```python
from build123d import *

# Parameters (mm, degrees)
SKETCH_R        = 6.65
PAD_DEPTH       = 10
SKETCH001_R     = 2.55
POCKET_DEPTH    = 10
SKETCH002_W     = 3.1
SKETCH002_H     = 15.6
PAD001_DEPTH    = 16
SKETCH003_R     = 2.55
POCKET001_DEPTH = 65.851


with BuildPart() as part:
    # Sketch → Pad (new body)
    with BuildSketch(Plane.XY):
        with BuildLine():
            Line((0, -15.35), (19.8, -15.35))
            ThreePointArc((19.8, -15.35), (28.780256, -11.630256), (32.5, -2.65))
            Line((32.5, -2.65), (32.5, 2.65))
            ThreePointArc((32.5, 2.65), (28.780256, 11.630256), (19.8, 15.35))
            Line((19.8, 15.35), (0, 15.35))
            Line((0, 15.35), (-17.35, 7.8))
            Line((-17.35, 7.8), (-33.35, 7.8))
            Line((-33.35, 7.8), (-33.35, -7.8))
            Line((-33.35, -7.8), (-17.35, -7.8))
            Line((-17.35, -7.8), (0, -15.35))
        make_face()
        with Locations((16.85, 0)):
            Circle(SKETCH_R, mode=Mode.SUBTRACT)
    extrude(amount=PAD_DEPTH)

    # Sketch001 (on Face3 of Pad) → Pocket (cut)
    with BuildSketch(Plane.YZ.offset(32.5)):
        with Locations((0, 5)):
            Circle(SKETCH001_R)
    extrude(amount=-POCKET_DEPTH, mode=Mode.SUBTRACT)

    # Sketch002 (on Face5 of Pocket) → Pad001 (join)
    with BuildSketch(Plane.XY.offset(10)):
        with Locations((-31.8, 0)):
            Rectangle(SKETCH002_W, SKETCH002_H)
        with Locations((-25.35, 0)):
            Rectangle(SKETCH002_W, SKETCH002_H)
        with Locations((-18.9, 0)):
            Rectangle(SKETCH002_W, SKETCH002_H)
    extrude(amount=PAD001_DEPTH)

    # Sketch003 (on Face24 of Pad001) → Pocket001 (cut, through all)
    with BuildSketch(Plane(origin=(-33.35, 0, 0), x_dir=(0, -1, 0), z_dir=(-1, 0, 0))):
        with Locations((0, 18.2)):
            Circle(SKETCH003_R)
        with BuildLine():
            ThreePointArc((7.8, 18.2), (0, 26), (-7.8, 18.2))
            Line((-7.8, 26.2), (-7.8, 18.2))
            Line((7.8, 26.2), (-7.8, 26.2))
            Line((7.8, 18.2), (7.8, 26.2))
        make_face()
    extrude(amount=-POCKET001_DEPTH, mode=Mode.SUBTRACT)


solid = part.part
```
Model file for the job. Use its own axes, mm. A direction names the side the tool comes from. Give positions to 0.01 mm unless a question says otherwise; leave off trailing zeros. Write each loop counter-clockwise with the first axis right and the second up, starting at its lowest first coordinate (ties: lowest second). Pieces come first, ordered by that corner, then holes. Notation, with made-up numbers: (84, 55.25) - (96, 55.25) arc R13 cw to (96, 79.25) - close; hole circle Ø2 at (-24, 87). An arc over 180 degrees is marked (long way). One line per question, with ' | ' between items. Start each with the question number.
(1) Slice it at B-B on y = 0. Give the number of separate pieces and of enclosed holes in the cut face, plus the area to 3 significant figures.
(2) Pin check, flat tips, straight feed: P1, Ø1, axis at x = -23, y = 1.5, coming from the +Z side; P2, Ø6.5, axis at y = 0, z = 18.2, coming from the +X side; P3, Ø3.5, axis at x = -28, y = -3.5, coming from the +Z side; P4, Ø2, axis at x = -0.5, z = 10, coming from the +Y side. Stop position of each tip, or through.
(3) Wall check: line 1 along X through (y, z) = (-4.5, 10.5); line 2 along Z through (x, y) = (-31.5, 0); line 3 along Y through (x, z) = (16.85, 2). Give the ranges that are in metal, low to high. Write a range as from..to.
(4) Slice it at D-D on y = 4. Write the cut outline in (x, z).
(5) Slice it at A-A on x = 16.85. Write the cut outline in (y, z).
(6) Two-plate mould, pull along X, no slides. Class faces 6 (the face through (-19, 0, 26)), 7 (the face through (-17.35, 2, 16)), 8 (the face through (-30.25, 2, 16)), 9 (the face through (-20.45, 2, 16)): +X half, -X half, draft (parallel to the pull), parting line (faces both ways), or undercut.
(7) 3-axis set-ups, long thin cutter, end or side, ignore diameter. For faces 1 (the face through (27.81, 1.37, 7.15)), 2 (the face through (-23.8, 2, 16)), 3 (the face through (7, 0, 10)), 4 (the face through (-25, -7.8, 7)), 5 (the face through (-25, 7.8, 7)): which of +Z, -Z, +X, -X, +Y, -Y reach the whole face in a straight line?
(8) Slice it at C-C on z = 12.75. Write the cut outline in (x, y), plus the area to 3 significant figures.
Results below:
1) separate pieces: 6 | enclosed holes: 0 | area: 581 mm^2
2) P1: z = 10 | P2: x = -17.35 | P3: z = 25.7 | P4: y = 15.35
3) line 1: -33.35..-30.25, -26.9..-23.8, -20.45..-17.35 | line 2: 0..15.65, 20.75..26 | line 3: -15.35..-6.65, 6.65..15.35
4) outline: (-33.35, 0) - (11.54, 0) - (11.54, 10) - (-17.35, 10) - (-17.35, 24.9) - (-20.45, 24.9) - (-20.45, 10) - (-23.8, 10) - (-23.8, 24.9) - (-26.9, 24.9) - (-26.9, 10) - (-30.25, 10) - (-30.25, 24.9) - (-33.35, 24.9) - close; (22.16, 0) - (32.43, 0) - (32.43, 10) - (22.16, 10) - close
5) outline: (-15.35, 0) - (-6.65, 0) - (-6.65, 10) - (-15.35, 10) - close; (6.65, 0) - (15.35, 0) - (15.35, 10) - (6.65, 10) - close
6) face 6: draft | face 7: +X half | face 8: undercut | face 9: undercut
7) face 1: +X | face 2: +Z, +Y, -Y | face 3: +Z, +X, +Y, -Y | face 4: +Z, -Z, -X, -Y | face 5: +Z, -Z, -X, +Y
8) outline: (-33.35, -7.8) - (-30.25, -7.8) - (-30.25, 7.8) - (-33.35, 7.8) - close; (-26.9, -7.8) - (-23.8, -7.8) - (-23.8, 7.8) - (-26.9, 7.8) - close; (-20.45, -7.8) - (-17.35, -7.8) - (-17.35, 7.8) - (-20.45, 7.8) - close | area: 145 mm^2
